Study the drawing (mm; zero at the part's minimum x, y, z) and answer. Round coordinates to 2 decimals unless told otherwise and drop trailing zeros. Loops run counter-clockwise (first coordinate to the right, second up) from the corner with the lowest first, then second, coordinate; pieces in that order, holes last. Notation, with made-up numbers: M 82.5,-7.75 L 112.5,-7.75 A20 cw 112.5,8.25 Z; hole C 63,48 d2. An arc over 180 degrees is marked long. Write each question's results on one line, items separated by ' | '.
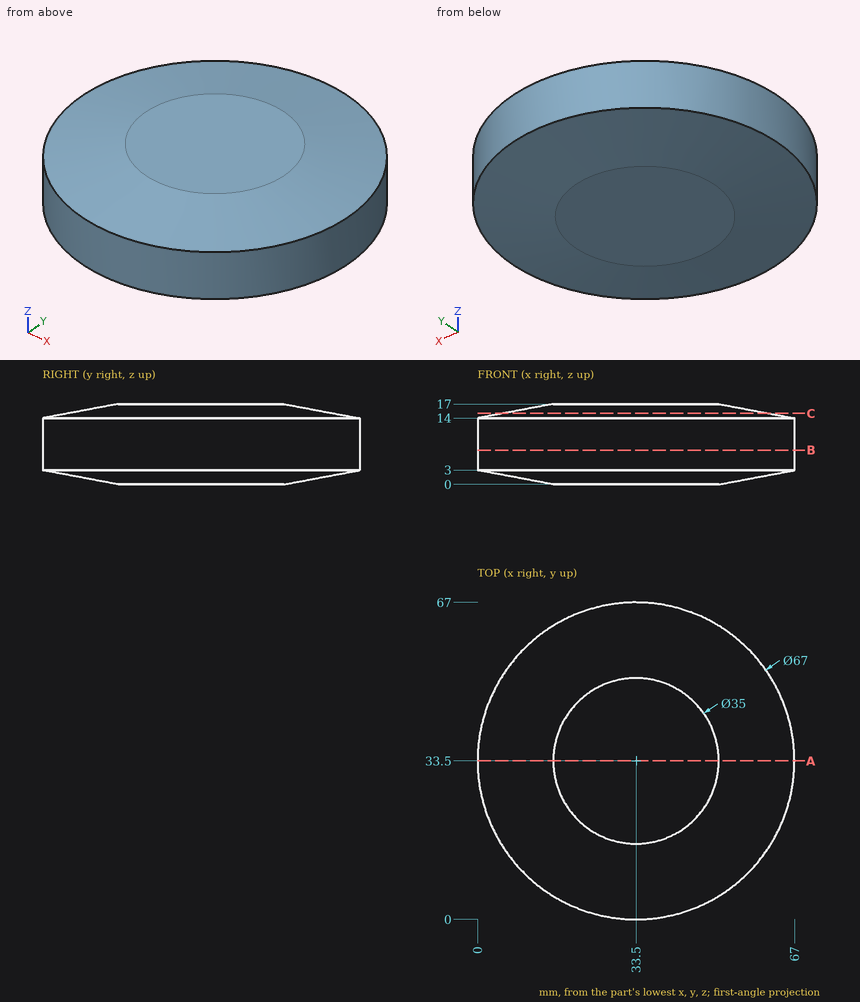
Item 1: The part is cut by section C-C (z = 15). Determine the outline of the cut face in (x, y).
Outcome:
outline: C 33.5,33.5 d56.33
Item 2: The part is cut by section B-B (z = 7.25). Determine the outline of the cut face in (x, y).
Outcome:
outline: C 33.5,33.5 d67
Item 3: The part is cut by section A-A (y = 33.5). Determine the outline of the cut face in (x, z).
Outcome:
outline: M 0,3 L 16,0 L 51,0 L 67,3 L 67,14 L 51,17 L 16,17 L 0,14 Z
Item 4: Straight lines are drawn through the part: line 1 (Y direction, x = 33, z = 11.25); line 2 (Y direction, x = 56, z = 4). For each, find the intervals that lie inside material, in ascending order.
Outcome:
line 1: y = 0 to 67 | line 2: y = 8.68 to 58.32
Item 5: Flat-ended cylindrical pins translate along their axes: pin 1 (8 mm diameter, centred on x = 32, z = 6, fed in from -Y); pin 2 (6 mm diameter, centred on x = 51, z = 9.5, fed in from -Y); pin 3 (1.5 mm diameter, centred on x = 44.5, y = 52, fed in from +Z). Find the tip coordinate at first contact, or state that the pin passes through.
Outcome:
pin 1: stops at y = 0 | pin 2: stops at y = 3.3 | pin 3: stops at z = 16.39
